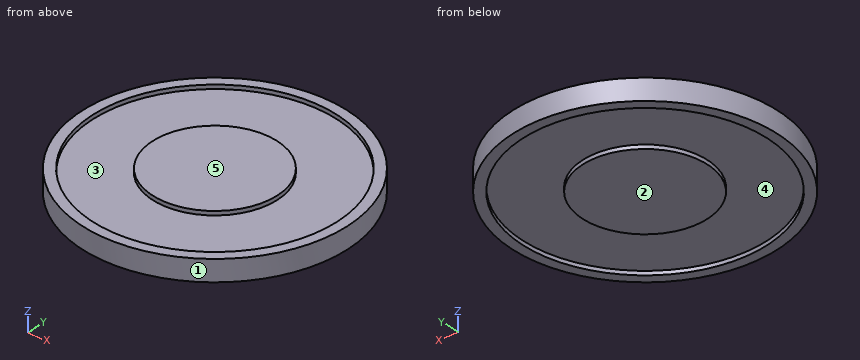
from build123d import *

# Parameters (mm, degrees)
SKETCH_R      = 32.5
SKETCH_R_2    = 12.8
PAD_DEPTH     = 3.2
SKETCH001_R   = 32.5
SKETCH001_R_2 = 30
SKETCH001_R_3 = 15.3
PAD001_DEPTH  = 1
SKETCH002_R   = 32.5
SKETCH002_R_2 = 30
SKETCH002_R_3 = 15.3
PAD002_DEPTH  = 1


with BuildPart() as part:
    # Sketch → Pad (new body)
    with BuildSketch(Plane.XY):
        Circle(SKETCH_R)
        Circle(SKETCH_R_2, mode=Mode.SUBTRACT)
    extrude(amount=PAD_DEPTH)

    # Sketch001 (on Face4 of Pad) → Pad001 (join)
    with BuildSketch(Plane.XY.offset(3.2)):
        Circle(SKETCH001_R)
        Circle(SKETCH001_R_2, mode=Mode.SUBTRACT)
        Circle(SKETCH001_R_3)
    extrude(amount=PAD001_DEPTH)

    # Sketch002 (on Face2 of Pad001) → Pad002 (join)
    with BuildSketch(Plane(origin=(0, 0, 0), x_dir=(1, 0, 0), z_dir=(0, 0, -1))):
        Circle(SKETCH002_R)
        Circle(SKETCH002_R_2, mode=Mode.SUBTRACT)
        Circle(SKETCH002_R_3)
    extrude(amount=PAD002_DEPTH)


solid = part.part
Work out the finished part from the listing and answer in its coordinate system (mm). Face numbers are marked on the shaded views. A direction names the side the tool comes from. Give positions to 0.01 mm unless a question says otherwise; leave off trailing zeros. Loops run counter-clockwise (first coordinate to the right, second up) from the corner with the lowest first, then second, coordinate; pieces in that order, holes last. Notation, with made-up numbers: (83.25, 8) -> (92.25, 8) arc R10 cw to (92.25, 12) -> close; hole circle Ø7 at (65, 86). An arc over 180 degrees is marked (long way). Use a Markdown table: item, result. Add a question column.
1) Each of these flat-tipped pins is pushed along its axis until it touches: P1, Ø1, axis at x = 17.5, y = -3, coming from the +Z side; P2, Ø2, axis at x = 2.5, y = 15.5, coming from the +Z side; P3, Ø1.5, axis at x = -26, z = 3.5, coming from the +Y side; P4, Ø3, axis at x = -24.5, z = 0.5, coming from the +Y side. Where does it stop, or does it pass through?
2) The part is cut by section D-D, the plane y = 28.5. Determine the outline of the cut face in (x, z).
3) For a pull along Y with two mould halves and no side action, classify the marked faces 1, 2 and 3 as +Y half, -Y half, draft (parallel to the pull), parting line (faces both ways), or undercut.
4) Which of the six approach directions +Z, -Z, +X, -X, +Y, -Y give full straight-line access (tool end or side, diameter ignored) to the marked faces 4 and 5?
5) The part is cut by section A-A, the plane x = 0. Determine the outline of the cut face in (y, z), plus the area to 3 significant figures.
6) The part is cut by section C-C, the plane z = 2.2. Determine the outline of the cut face in (x, y), plus the area to 3 significant figures.
7) Consider line 1 along X through (y, z) = (0, -0.55); line 2 along Y through (x, z) = (0, 2.5); line 3 along Z through (x, y) = (11.5, 2.5). Determine where each line is inside the solid, lowest interval first.
Reported:
| question | item | result |
|---|---|---|
| 1 | P1 | stops at z = 3.2 |
| 1 | P2 | stops at z = 4.2 |
| 1 | P3 | stops at y = 20.46 |
| 1 | P4 | stops at y = 22.96 |
| 2 | outline | (-15.62, -1) -> (-9.37, -1) -> (-9.37, 0) -> (9.37, 0) -> (9.37, -1) -> (15.62, -1) -> (15.62, 4.2) -> (9.37, 4.2) -> (9.37, 3.2) -> (-9.37, 3.2) -> (-9.37, 4.2) -> (-15.62, 4.2) -> close |
| 3 | face 1 | parting line |
| 3 | face 2 | draft |
| 3 | face 3 | undercut |
| 4 | face 4 | -Z |
| 4 | face 5 | +Z, +X, -X, +Y, -Y |
| 5 | outline | (-32.5, -1) -> (-30, -1) -> (-30, 0) -> (-15.3, 0) -> (-15.3, -1) -> (15.3, -1) -> (15.3, 0) -> (30, 0) -> (30, -1) -> (32.5, -1) -> (32.5, 4.2) -> (30, 4.2) -> (30, 3.2) -> (15.3, 3.2) -> (15.3, 4.2) -> (-15.3, 4.2) -> (-15.3, 3.2) -> (-30, 3.2) -> (-30, 4.2) -> (-32.5, 4.2) -> close; hole (-12.8, 0) -> (12.8, 0) -> (12.8, 3.2) -> (-12.8, 3.2) -> close |
| 5 | area | 197 mm^2 |
| 6 | outline | circle Ø65 at (0, 0); hole circle Ø25.6 at (0, 0) |
| 6 | area | 2,800 mm^2 |
| 7 | line 1 | x = -32.5 to -30, -15.3 to 15.3, 30 to 32.5 |
| 7 | line 2 | y = -32.5 to -12.8, 12.8 to 32.5 |
| 7 | line 3 | z = -1 to 0, 3.2 to 4.2 |
